Design review of the part built by this model. Coordinates are the model's own, in mm. Give positions to 0.01 mm unless a question says otherwise; leave off trailing zeros. Order: outer loops, then holes, each group sorted by start corner. A loop starts at its lowest first (then second) coordinate and runs counter-clockwise, first axis right, second up. Notation, with made-up numbers: (61, 43) -> (103, 43) arc R23 ccw to (103, 60) -> close; hole circle Ø3 at (81, -27.5). An arc over 180 degrees is marked (long way). One line per item, written item: value. Start each with the question number.
1) Consider section A-A (z = 1017). State the section outline as (x, y) points.
2) Wall thickness on line 1 along Y through (x, z) = (5, 732); line 2 along X through (y, z) = (2, 356.5); line 3 along Y through (x, z) = (-10, 1155.5): over which ranges is each line inside the solid? List them lowest first. Write a range as from..to.
3) Consider section B-B (z = 149). State the section outline as (x, y) points, plus the area to 3 significant figures.
4) For pin 1 (12 mm diameter, centred on x = -1, z = 817.5, fed in from -Y); pin 2 (6 mm diameter, centred on y = -31, z = 644.5, fed in from +X); pin 3 (3 mm diameter, centred on x = 30.5, z = 652, fed in from -Y), all flat-tipped, find the tip position at first contact; note any pin that passes through.
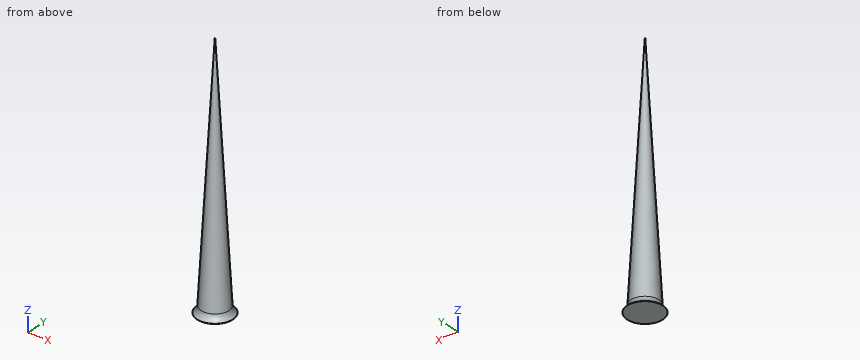
from build123d import *

# Parameters (mm, degrees)
F0_R     = 85
F2_R     = 0.5
F4_R     = 105.9677495378
F5_DEPTH = 1


# Not quite as in the source:
# - a fillet or chamfer that OpenCascade refuses, or shapes differently, is made with other operations: its cross-section is extruded or revolved along the edge and cut away or added


with BuildPart() as f3:
    # F0 (on Top) → F3 section 0
    with BuildSketch(Plane.XY):
        Circle(F0_R)
    # F2 (on offset) → F3 section 1
    with BuildSketch(Plane.XY.offset(1500)):
        Circle(F2_R)
    loft()

    # F4 (on Top) → F5 (join)
    with BuildSketch(Plane.XY):
        Circle(F4_R)
    extrude(amount=F5_DEPTH)

    # F6: fillet of radius 50 on 1 edges, made by hand


with BuildPart() as f6_tool2:
    # F6_s3 → F6_t4 (revolve)
    with BuildSketch(Plane.XZ):
        with BuildLine():
            ThreePointArc((105.9675361519, 0.9996616711), (89.555381413, 17.9202187852), (82.7192415892, 40.4797238448))
            Line((82.7192415892, 40.4797238448), (77.7270102291, 40.1984948115))
            ThreePointArc((77.7270102291, 40.1984948115), (78.8394224512, 20.458644138), (79.9514353065, 0.7187709667))
            Line((79.9514353065, 0.7187709667), (84.9436666667, -4.0001463701))
            ThreePointArc((84.9436666667, -4.0001463701), (95.4556014093, -4.0001463701), (103.300134248, -3.2295735796))
            Line((103.300134248, -3.2295735796), (105.9675361519, 0.9996616711))
        make_face()
    revolve(axis=Axis((0, 0, 1), (0, 0, 1)))

    split(bisect_by=Plane.XY, keep=Keep.TOP)


with BuildPart() as f3_1:
    add(f3.part)

    # F6_t1: union F6_tool2
    add(f6_tool2.part)


solid = f3_1.part
Checked values:
1. outline: circle Ø55.42 at (0, 0)
2. line 1: y = -43.48..43.48
2. line 2: x = -64.89..64.89
2. line 3: y = -17.21..17.21
3. outline: circle Ø153.21 at (0, 0)
3. area: 18,400 mm^2
4. pin 1: stops at y = -39.28
4. pin 2: stops at x = 39.85
4. pin 3: stops at y = -38.59
